The listing builds one solid part. Answer for the finished solid, in the listing's coordinates (mm). A direction names the side the tool comes from. Coordinates: 2 decimals unless noted, no trailing zeros. Loops run counter-clockwise (first coordinate to the right, second up) from the corner with the lowest first, then second, coordinate; pieces in that order, holes last. Notation, with made-up numbers: (3.5, 20.25) - (12.5, 20.25) arc R18 ccw to (12.5, 47.25) - close; hole circle Ø11 at (29.25, 64.25). An arc over 180 degrees is marked (long way). One line per question, with ' | ' between items.
from build123d import *

# Parameters (mm, degrees)
SKETCH1_R           = 1.5
BOSS_EXTRUDE1_DEPTH = 3


with BuildPart() as part:
    # Sketch1 → Boss-Extrude1 (new body)
    with BuildSketch(Plane.XY):
        with BuildLine():
            Line((-0.6125, 6.973151637), (-40.30625, 3.486575818))
            ThreePointArc((-40.30625, 3.486575818), (-43.5, 0), (-40.30625, -3.486575818))
            Line((-40.30625, -3.486575818), (-0.6125, -6.973151637))
            ThreePointArc((-0.6125, -6.973151637), (7, 0), (-0.6125, 6.973151637))
        make_face()
        with Locations((-40, 0)):
            Circle(SKETCH1_R, mode=Mode.SUBTRACT)
        with BuildLine():
            ThreePointArc((-3.305072464, -0.989442272), (-3.377344208, -0.997357075), (-3.45, -1))
            Line((-3.45, -1), (-15.45, -1))
            ThreePointArc((-15.45, -1), (-16.45, 0), (-15.45, 1))
            Line((-15.45, 1), (-3.45, 1))
            ThreePointArc((-3.45, 1), (-3.377344208, 0.997357075), (-3.305072464, 0.989442272))
            ThreePointArc((-3.305072464, 0.989442272), (0.5, 3.413575838), (3.45, 0))
            ThreePointArc((3.45, 0), (0.5, -3.413575838), (-3.305072464, -0.989442272))
        make_face(mode=Mode.SUBTRACT)
    extrude(amount=BOSS_EXTRUDE1_DEPTH)


solid = part.part
Item 1: Find section A-A, the plane x = 0. Write down the section's boundary in (y, z).
Taken from the geometry:
outline: (-7, 0) - (-3.45, 0) - (-3.45, 3) - (-7, 3) - close; (3.45, 0) - (7, 0) - (7, 3) - (3.45, 3) - close
Item 2: Find the intervals of material crossed by line 1 (Y direction, x = -40, z = 2.35); line 2 (Y direction, x = 0, z = 1); line 3 (Y direction, x = -22, z = 1.05), in increasing order. Write a range as [from, to].
Taken from the geometry:
line 1: y = [-3.51, -1.5], [1.5, 3.51] | line 2: y = [-7, -3.45], [3.45, 7] | line 3: y = [-5.09, 5.09]
Item 3: The mould has two halves that part along X. Classify faces 3 (the face through (-19, 0, 0)), 4 (the face through (-20.737, -5.205, 1.479)), 5 (the face through (-41.5, 0.07, 1.48)): pulls with the +X half, pulls with the -X half, needs draft (parallel to the pull), parting line crosses it, or undercut.
Taken from the geometry:
face 3: needs draft | face 4: pulls with the -X half | face 5: undercut
Item 4: Which of the six approach directions +Z, -Z, +X, -X, +Y, -Y give full straight-line access (tool end or side, diameter ignored) to faces 1 (the face through (-19, 0, 3)), 2 (the face through (-16.45, -0.02, 1.48))?
Taken from the geometry:
face 1: +Z, +X, -X, +Y, -Y | face 2: +Z, -Z
Item 5: Find section B-B, the plane z = 2.1. Write down the section's boundary in (x, y), plus the area to 3 significant figures.
Taken from the geometry:
outline: (-40.31, -3.49) - (-0.61, -6.97) arc R7 ccw (long way) to (-0.61, 6.97) - (-40.31, 3.49) arc R3.5 ccw to start; hole circle Ø3 at (-40, 0); hole (-15.45, -1) - (-3.45, -1) arc R1 ccw to (-3.31, -0.99) arc R3.45 ccw (long way) to (-3.31, 0.99) arc R1 ccw to (-3.45, 1) - (-15.45, 1) arc R1 ccw to start | area: 448 mm2
Item 6: Each of these flat-tipped pins is pushed along its axis until it touches: pin 1 Ø1 at (y, z) = (-2, 1) entering from -X; pin 2 Ø1.5 at (x, z) = (-28, 1.5) entering from -Y; pin 3 Ø1.5 at (x, z) = (-7.5, 2) entering from -Y. Where does it stop, or does it pass through?
Taken from the geometry:
pin 1: stops at x = -43.16 | pin 2: stops at y = -4.63 | pin 3: stops at y = -6.43
Item 7: Find section D-D, the plane y = 5. Write down the section's boundary in (x, z).
Taken from the geometry:
outline: (-23.08, 0) - (4.9, 0) - (4.9, 3) - (-23.08, 3) - close
Item 8: Find section C-C, the plane y = -2.25. Write down the section's boundary in (x, z), plus the area to 3 significant figures.
Taken from the geometry:
outline: (-42.68, 0) - (-2.62, 0) - (-2.62, 3) - (-42.68, 3) - close; (2.62, 0) - (6.63, 0) - (6.63, 3) - (2.62, 3) - close | area: 132 mm2
